Read the model definition and answer for the solid it produces. Units are mm, in the model's axes. Face numbers are marked on the shaded views. A direction names the side the tool comes from. Round coordinates to 2 decimals unless told otherwise and drop trailing zeros. Write each loop counter-clockwise with the first axis right and the second up, starting at its lowest first coordinate (ties: lowest second). Pieces come first, ordered by that corner, then holes. Notation, with made-up numbers: (5, 74) - (40, 74) arc R31 ccw to (40, 100) - close; hole circle Ø10 at (65.5, -38.75). An arc over 180 degrees is marked (long way). Answer as CSV lines item,"result". Start each with the question number.
1) Each of these flat-tipped pins is pushed along its axis until it touches: pin 1 (4 mm diameter, centred on x = 2.5, z = -113, fed in from +Y); pin 2 (3 mm diameter, centred on x = -19.5, z = -141.5, fed in from -Y); pin 3 (12 mm diameter, centred on x = -14, y = 101.5, fed in from +Z). Where does it stop, or does it pass through?
2) For a pull along X with two mould halves and no side action, classify the marked faces 4, 5 and 6 as +X half, -X half, draft (parallel to the pull), parting line (faces both ways), or undercut.
3) Find section D-D on z = -165.5. Determine the outline of the cut face in (x, y) (3 decimals), then the cut area to 3 significant figures.
4) Find section B-B on z = -52.5. Determine the outline of the cut face in (x, y).
5) Find section C-C on y = 115.5. Determine the outline of the cut face in (x, z), then the cut area to 3 significant figures.
6) Find section A-A on x = 0. Determine the outline of the cut face in (y, z).
7) Which of the six approach directions +Z, -Z, +X, -X, +Y, -Y give full straight-line access (tool end or side, diameter ignored) to the marked faces 1, 2 and 3?
8) Consider line 1 along Z through (x, y) = (-48.5, 134); line 2 along X through (y, z) = (115.5, -158); line 3 along Y through (x, z) = (4, -73.5). Determine where each line is inside the solid, lowest interval first.
Autodesk Inventor part; units mm, degrees
ref_plane "YZ Plane" through (0, 0, 0) normal (1, 0, 0) x (0, 1, 0)
ref_plane "XZ Plane" through (0, 0, 0) normal (0, 1, 0) x (-1, 0, 0)
ref_plane "XY Plane" through (0, 0, 0) normal (0, 0, 1) x (1, 0, 0)
sketch "Sketch1" plane through (0, 0, 0) normal (0, 0, 1) x (1, 0, 0)
  point P0 (0, 0)
sketch "Sketch2" plane through (0, 0, 0) normal (0, 0, 1) x (1, 0, 0)
  line L0 (-50, -25) -> (50, -25)
  line L1 (50, -25) -> (50, 25)
  line L2 (50, 25) -> (-50, 25)
  line L3 (-50, 25) -> (-50, -25)
  line L4 (-50, -25) -> (50, 25) construction
  line L5 (50, -25) -> (-50, 25) construction
  line L6 (-55, -30) -> (55, -30)
  line L7 (55, -30) -> (55, 30)
  line L8 (55, 30) -> (-55, 30)
  line L9 (-55, 30) -> (-55, -30)
  line L10 (-55, -30) -> (55, 30) construction
  line L11 (55, -30) -> (-55, 30) construction
  point P0 (0, 0)
  dimension "d0" = 100
  dimension "d1" = 50
  dimension "d2" = 110
  dimension "d3" = 60
sketch "Sketch3" plane through (0, 0, 0) normal (1, 0, 0) x (0, 1, 0)
  line L0 (0, 0) -> (0, -75)
  arc A0 (0, -75) -> (100, -175) centre (100, -75) ccw
  line L1 (100, -75) -> (100, -175) construction
  line L2 (100, -75) -> (0, -75) construction
  line L3 (100, -175) -> (150, -175)
sweep "Sweep1" add profiles "Sketch2" path "Sketch3"
properties part number "RecTubeNew"
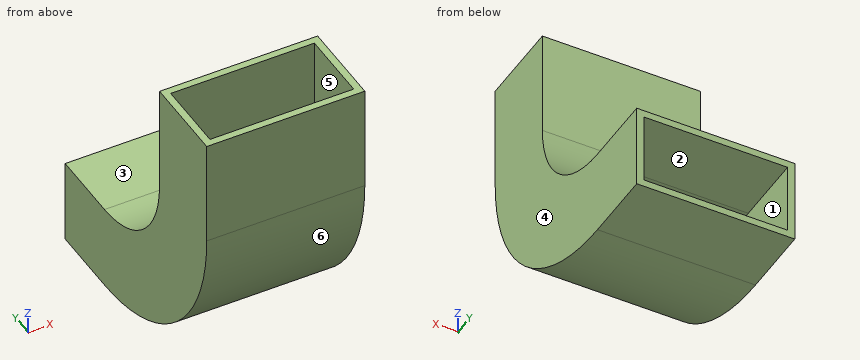
Check values:
1,pin 1,"stops at y = 42.55"
1,pin 2,"stops at y = -12.58"
1,pin 3,"stops at z = -144.86"
2,face 4,"+X half"
2,face 5,"undercut"
2,face 6,"draft"
3,outline,"(-55, 6.674) - (55, 6.674) - (55, 150) - (50, 150) - (50, 13.775) - (-50, 13.775) - (-50, 150) - (-55, 150) - close"
3,area,"2,140 mm^2"
4,outline,"(-55, -30) - (55, -30) - (55, 30) - (-55, 30) - close; hole (-50, -25) - (50, -25) - (50, 25) - (-50, 25) - close"
5,outline,"(-55, -205) - (55, -205) - (55, -145) - (-55, -145) - close; hole (-50, -200) - (50, -200) - (50, -150) - (-50, -150) - close"
5,area,"1,600 mm^2"
6,outline,"(-30, -75) arc R130 ccw to (100, -205) - (150, -205) - (150, -200) - (100, -200) arc R125 cw to (-25, -75) - (-25, 0) - (-30, 0) - close; (25, -75) arc R75 ccw to (100, -150) - (150, -150) - (150, -145) - (100, -145) arc R70 cw to (30, -75) - (30, 0) - (25, 0) - close"
7,face 1,"none"
7,face 2,"+Y"
7,face 3,"+Z, +X, -X, +Y"
8,line 1,"z = -205 to -200, -150 to -145"
8,line 2,"x = -55 to -50, 50 to 55"
8,line 3,"y = -30 to -25, 25 to 30"
